from build123d import *

# Parameters (mm, degrees)
SKETCH2_R          = 1.5
CUT_EXTRUDE1_DEPTH = 3
SKETCH3_R          = 1.5
CUT_EXTRUDE2_DEPTH = 2.8


with BuildPart() as part:
    # Sketch1 → Revolve1 (revolve)
    with BuildSketch(Plane.XY):
        with BuildLine():
            Line((0, 0), (11.8, 0))
            Line((11.8, 0), (11.8, 0.7))
            Line((11.8, 0.7), (12.4, 0.7))
            ThreePointArc((12.4, 0.7), (12.965636633, 2.38480236), (14, 3.83))
            Line((14, 3.83), (14, 4.5))
            Line((14, 4.5), (13.5, 4.5))
            Line((13.5, 4.5), (13.5, 5.3))
            Line((13.5, 5.3), (14, 5.3))
            Line((14, 5.3), (14, 6.1))
            Line((14, 6.1), (2, 6.1))
            Line((2, 6.1), (2, 6.6))
            Line((2, 6.6), (14, 6.6))
            Line((14, 6.6), (14, 17.7))
            Line((14, 17.7), (13.6, 17.7))
            Line((13.6, 17.7), (13.6, 18.4))
            Line((13.6, 18.4), (14, 18.4))
            Line((14, 18.4), (14, 19))
            Line((14, 19), (12.5, 22))
            Line((12.5, 22), (2, 22))
            Line((2, 22), (2, 37))
            Line((2, 37), (0, 37))
            Line((0, 37), (0, 0))
        make_face()
    revolve(axis=Axis((0, 37, 0), (0, -1, 0)))

    # Sketch2 → Cut-Extrude1 (cut)
    with BuildSketch(Plane.XZ):
        with Locations((0, 8)):
            Circle(SKETCH2_R)
        with Locations((9.5, 0)):
            Circle(SKETCH2_R)
        with Locations((0, -8)):
            Circle(SKETCH2_R)
        with Locations((-9.5, 0)):
            Circle(SKETCH2_R)
    extrude(amount=-CUT_EXTRUDE1_DEPTH, mode=Mode.SUBTRACT)

    # Sketch3 → Cut-Extrude2 (cut)
    with BuildSketch(Plane(origin=(0, 22, 0), x_dir=(1, 0, 0), z_dir=(0, 1, 0))):
        with Locations((0, 10)):
            Circle(SKETCH3_R)
        with Locations((10, 0)):
            Circle(SKETCH3_R)
        with Locations((0, -10)):
            Circle(SKETCH3_R)
        with Locations((-10, 0)):
            Circle(SKETCH3_R)
    extrude(amount=-CUT_EXTRUDE2_DEPTH, mode=Mode.SUBTRACT)


solid = part.part
Check sheet for the modelled part. Datum: model origin and axes. Units: mm. A direction names the side the tool comes from. Coordinates: 2 decimals unless noted, no trailing zeros. Write each loop counter-clockwise with the first axis right and the second up, starting at its lowest first coordinate (ties: lowest second). Pieces come first, ordered by that corner, then holes. Notation, with made-up numbers: M 0.5,-0.5 L 27.5,-0.5 A6 cw 27.5,6.5 Z; hole C 18,70.25 d5. An arc over 180 degrees is marked long. Answer as CSV lines item,"result".
Q1. Material ranges on probe 1 along Y at (x, z) = (7.75, -1); probe 2 along Z at (x, y) = (0, 20.1); probe 3 along Z at (x, y) = (0, 2.3), recorded low to high. Write a range as from..to.
Check result:
probe 1,"0..6.1, 6.6..22"
probe 2,"-13.45..-11.5, -8.5..8.5, 11.5..13.45"
probe 3,"-12.92..-9.5, -6.5..6.5, 9.5..12.92"
Q2. Mould release check, pull along X, two halves, no side actions. Record for faces 1 (the face through (-11, 0.7, -5)), 2 (the face through (12.932, 5.706, -5.362)), 3 (the face through (-0.325, 20.62, 11.464)), 4 (the face through (9, 3, 0)): released by +X, released by -X, zero draft, split by the parting line, or undercut.
Check result:
face 1,"zero draft"
face 2,"split by the parting line"
face 3,"undercut"
face 4,"undercut"
Q3. Cross-section at A-A (y = 33.5). Record the boundary of the cut face in (x, z), then the cut area to 3 significant figures.
Check result:
outline,"C 0,0 d4"
area,"12.6 mm^2"
Q4. Cross-section at B-B (y = 10). Record the boundary of the cut face in (x, z), then the cut area to 3 significant figures.
Check result:
outline,"C 0,0 d28"
area,"616 mm^2"
Q5. Go/stop test with flat-tipped pins: pin 1 (6 mm diameter, centred on x = 3, y = 12.5, fed in from +Z); pin 2 (3.5 mm diameter, centred on x = 10, z = 0, fed in from +Y); pin 3 (2.5 mm diameter, centred on x = 9.5, z = 0, fed in from -Y); pin 4 (2.5 mm diameter, centred on x = 0, z = -10, fed in from +Y). Record where each tip stops, or that it passes through.
Check result:
pin 1,"z = 14"
pin 2,"y = 22"
pin 3,"y = 3"
pin 4,"y = 19.2"
Q6. Set-up check for faces 5 (the face through (-10, 3, 0)), 6 (the face through (0, 19.2, 10)), 7 (the face through (12.932, 4.17, -5.362)): record each of +Z, -Z, +X, -X, +Y, -Y from which the full face is reachable in a straight line by a thin tool's end or side.
Check result:
face 5,"-Y"
face 6,"+Y"
face 7,"+Y, -Y"
